Geometry check sheet. Reference: the model listing, model coordinates, mm. A direction names the side the tool comes from. Coordinates: 2 decimals unless noted, no trailing zeros. Write each loop counter-clockwise with the first axis right and the second up, starting at its lowest first coordinate (ties: lowest second). Pieces come first, ordered by that corner, then holes. Notation, with made-up numbers: (43.5, 88.5) -> (56.5, 88.5) arc R27 cw to (56.5, 125.5) -> close; hole circle Ø1 at (52, 29). An arc over 180 degrees is marked (long way). Answer in a Markdown table with one row per item. Add a question column.
1. Depth check by flat-ended pin: P1, Ø4, axis at x = -73.5, z = 68, coming from the +Y side; P2, Ø8, axis at x = -63.5, y = 86.5, coming from the -Z side; P3, Ø2, axis at x = 88, y = 75, coming from the +Z side. Enter the tip coordinate at first touch or a pass-through.
2. Scan lines: L1, parallel to Z at x = -88.5, y = 61; L2, parallel to Y at x = -44.5, z = 71. Record each from-to range of solid material in increasing order. Write a range as from..to.
3. Cross-section at D-D on z = 46.5. Record the cut outline in (x, y), and give its area (3 significant figures).
4. Cross-section at B-B on x = 0. Record the cut outline in (y, z), and give its area (4 significant figures).
5. Set-up check for faces 4 (the flat face through (-1, -5, 1)), 5 (the flat face through (-14, 51, -12.5)): record each of +Z, -Z, +X, -X, +Y, -Y from which the full face is reachable in a straight line by a thin tool's end or side.
6. Cross-section at A-A on x = 50.5. Record the cut outline in (y, z), and give its area (3 significant figures).
7. Mould release check, pull along Y, two halves, no side actions. Record for faces 1 (the flat face through (14, 100, 0)), 2 (the flat face through (66.906, 32.115, 0.175)), 3 (the flat face through (-14, 51, 12.5)): pulls with the +Y half, pulls with the -Y half, needs draft (parallel to the pull), parting line crosses it, or undercut.
8. Cross-section at C-C on y = 39. Record the cut outline in (x, z), and give its area (3 significant figures).
```python
from build123d import *

# Parameters (mm, degrees)
F0_R     = 100
F1_DEPTH = 5
F3_DEPTH = 12.5


with BuildPart() as f1:
    # F0 (on Front) → F1 (new body, symmetric)
    with BuildSketch(Plane.XZ):
        Circle(F0_R)
    extrude(amount=F1_DEPTH, both=True)

    # F2 (on Top) → F3 (join, symmetric)
    with BuildSketch(Plane.XY):
        Polygon((-100, 0), (0, 0), (125, 60), (125, 100), (-100, 100), align=None)
    extrude(amount=F3_DEPTH, both=True)


solid = f1.part
```
Results found:
| question | item | result |
|---|---|---|
| 1 | P1 | stops at y = 5 |
| 1 | P2 | stops at z = -12.5 |
| 1 | P3 | stops at z = 12.5 |
| 2 | L1 | z = -12.5..12.5 |
| 2 | L2 | y = -5..5 |
| 3 | outline | (-88.53, -5) -> (88.53, -5) -> (88.53, 5) -> (-88.53, 5) -> close |
| 3 | area | 1,770 mm^2 |
| 4 | outline | (-5, -100) -> (5, -100) -> (5, -12.5) -> (100, -12.5) -> (100, 12.5) -> (5, 12.5) -> (5, 100) -> (-5, 100) -> close |
| 4 | area | 4,375 mm^2 |
| 5 | face 4 | +Z, -Z, +X, -X, -Y |
| 5 | face 5 | -Z, +X, -X, +Y |
| 6 | outline | (-5, -86.31) -> (5, -86.31) -> (5, 86.31) -> (-5, 86.31) -> close; (24.24, -12.5) -> (100, -12.5) -> (100, 12.5) -> (24.24, 12.5) -> close |
| 6 | area | 3,620 mm^2 |
| 7 | face 1 | pulls with the +Y half |
| 7 | face 2 | undercut |
| 7 | face 3 | needs draft |
| 8 | outline | (-100, -12.5) -> (81.25, -12.5) -> (81.25, 12.5) -> (-100, 12.5) -> close |
| 8 | area | 4,530 mm^2 |
